```python
from build123d import *

# Parameters (mm, degrees)
SKETCH1_R           = 45
BOSS_EXTRUDE1_DEPTH = 15
SKETCH2_R           = 43.5
CUT_EXTRUDE1_DEPTH  = 4.8
SKETCH3_R           = 43.487927738
SKETCH3_R_2         = 38.8
CUT_EXTRUDE2_DEPTH  = 5.4


with BuildPart() as part:
    # Sketch1 → Boss-Extrude1 (new body)
    with BuildSketch(Plane(origin=(0, 0, 0), x_dir=(1, 0, 0), z_dir=(0, 1, 0))):
        with Locations(Location((0, 0, 0), (0, 0, 270))):
            Circle(SKETCH1_R)
    extrude(amount=BOSS_EXTRUDE1_DEPTH)

    # Sketch2 → Cut-Extrude1 (cut)
    with BuildSketch(Plane(origin=(0, 15, 0), x_dir=(1, 0, 0), z_dir=(0, 1, 0))):
        with Locations(Location((0, 0, 0), (0, 0, 270))):
            Circle(SKETCH2_R)
    extrude(amount=-CUT_EXTRUDE1_DEPTH, mode=Mode.SUBTRACT)

    # Sketch3 → Cut-Extrude2 (cut)
    with BuildSketch(Plane(origin=(0, 10.2, 0), x_dir=(1, 0, 0), z_dir=(0, 1, 0))):
        with Locations(Location((0, 0, 0), (0, 0, 270))):
            Circle(SKETCH3_R)
        with Locations(Location((0, 0, 0), (0, 0, 270))):
            Circle(SKETCH3_R_2, mode=Mode.SUBTRACT)
    extrude(amount=-CUT_EXTRUDE2_DEPTH, mode=Mode.SUBTRACT)


solid = part.part
```
Source: CAD feature listing. Evaluate the final solid. Frame: model axes, mm. A direction names the side the tool comes from. Coordinates: 2 decimals unless noted, no trailing zeros. Loops run counter-clockwise (first coordinate to the right, second up) from the corner with the lowest first, then second, coordinate; pieces in that order, holes last. Notation, with made-up numbers: M -4,-16 L 15,-16 A24 cw 15,23 Z; hole C -28.75,44 d2. An arc over 180 degrees is marked long. Use CSV: the item, a comma, the result in double quotes.
(1) Reachability of faces 4 (the face through (11.65, 7.54, 37.01)), 5 (the face through (24, 15, -37)) from +Z, -Z, +X, -X, +Y, -Y: full face, straight path, thin tool, end or side. Return the list, or none.
Answers follow:
face 4,"+Y"
face 5,"+Z, -Z, +X, -X, +Y"
(2) Cut plane C-C on y = 7.5. Return loops of the section in (x, z).
Answers follow:
outline,"C 0,0 d90; C 0,0 d77.6; hole C 0,0 d86.98"
(3) Cut plane D-D on y = 1.5. Return loops of the section in (x, z), and give its area (3 significant figures).
Answers follow:
outline,"C 0,0 d90"
area,"6,360 mm²"
(4) Contact query for flat-ended pins moving along their axis: pin 1 (1.5 mm diameter, centred on x = -24.5, z = -17, fed in from +Y); pin 2 (2 mm diameter, centred on y = 8, z = -15.5, fed in from -X); pin 3 (5 mm diameter, centred on x = 10.5, y = 3.5, fed in from +Z). Output: stop coordinate, or through.
Answers follow:
pin 1,"y = 10.2"
pin 2,"x = -42.6"
pin 3,"z = 44.28"
(5) Draft query along X for faces 1 (the face through (1, 0, -1)), 2 (the face through (1, 10.2, -1)), 3 (the face through (-17.235, 7.395, 41.569)). Return one class per face: pulls with the +X half, pulls with the -X half, needs draft (parallel to the pull), parting line crosses it, or undercut.
Answers follow:
face 1,"needs draft"
face 2,"undercut"
face 3,"parting line crosses it"
(6) Line query: line 1 (X direction, y = 6.45, z = 0); line 2 (Z direction, x = 12, y = 9.5); line 3 (Z direction, x = 29.5, y = 8.75). Output: solid intervals per line, ascending. Write a range as [from, to].
Answers follow:
line 1,"[-45, -43.49], [-38.8, 38.8], [43.49, 45]"
line 2,"[-43.37, -41.8], [-36.9, 36.9], [41.8, 43.37]"
line 3,"[-33.98, -31.95], [-25.2, 25.2], [31.95, 33.98]"
